from build123d import *

# Parameters (mm, degrees)
SKETCH1_R           = 22
SKETCH1_R_2         = 20
BOSS_EXTRUDE1_DEPTH = 10
BOSS_EXTRUDE2_START = 100
SKETCH1_3_R         = 22
SKETCH1_3_R_2       = 20
BOSS_EXTRUDE2_DEPTH = 100
FILLET1_R           = 5
FILLET2_R           = 5
BOSS_EXTRUDE3_DEPTH = 2
CHAMFER1_SIZE       = 2.5
CHAMFER1_SIZE_2     = 6.868693549


with BuildPart() as part:
    # Sketch1 → Boss-Extrude1 (new body)
    # profile 1 of 2: a face of its own
    with BuildSketch(Plane(origin=(0, 0, 0), x_dir=(1, 0, 0), z_dir=(0, 1, 0))):
        with Locations(Location((0, 0, 0), (0, 0, 270))):
            Circle(SKETCH1_R)
        Circle(SKETCH1_R_2, mode=Mode.SUBTRACT)
    # profile 2 of 2: a face of its own
    with BuildSketch(Plane(origin=(0, 0, 0), x_dir=(1, 0, 0), z_dir=(0, 1, 0))):
        Circle(SKETCH1_R_2)
    extrude(amount=-BOSS_EXTRUDE1_DEPTH)

    # Sketch1<3> → Boss-Extrude2 (add)
    with BuildSketch(Plane(origin=(0, 0, 0), x_dir=(1, 0, 0), z_dir=(0, 1, 0)).offset(BOSS_EXTRUDE2_START)):
        with Locations(Location((0, 0, 0), (0, 0, 270))):
            Circle(SKETCH1_3_R)
        with Locations(Location((0, 0, 0), (0, 0, 270))):
            Circle(SKETCH1_3_R_2, mode=Mode.SUBTRACT)
    extrude(amount=-BOSS_EXTRUDE2_DEPTH)

    # Fillet1
    fillet1_edges = [part.edges().sort_by_distance(p)[0] for p in [
        (0, 0, -20),
    ]]
    fillet(fillet1_edges, radius=FILLET1_R)

    # Fillet2
    fillet2_edges = [part.edges().sort_by_distance(p)[0] for p in [
        (0, -10, -22),
    ]]
    fillet(fillet2_edges, radius=FILLET2_R)

    # Sketch2 → Boss-Extrude3 (add)
    with BuildSketch(Plane.XZ.offset(10)):
        with BuildLine():
            ThreePointArc((2.165063509, 10.75), (0, 12), (-2.165063509, 10.75))
            Line((-2.165063509, 10.75), (-2.5, 10.169872981))
            Line((-2.5, 10.169872981), (-2.5, 0))
            ThreePointArc((-2.5, 0), (0, -2.5), (2.5, 0))
            Line((2.5, 0), (2.5, 10.169872981))
            Line((2.5, 10.169872981), (2.165063509, 10.75))
        make_face()
        with BuildLine():
            ThreePointArc((-2.165063509, -4.75), (-2.5, -6), (-2.165063509, -7.25))
            Line((-2.165063509, -7.25), (2.165063509, -7.25))
            ThreePointArc((2.165063509, -7.25), (2.5, -6), (2.165063509, -4.75))
            Line((2.165063509, -4.75), (-2.165063509, -4.75))
        make_face()
    extrude(amount=BOSS_EXTRUDE3_DEPTH)

    # Chamfer1
    # the kernel refuses this chamfer: 6.868693549, 2.5 mm, written as the material it takes off along each edge
    with BuildSketch(Plane(origin=(0, 100, 0), x_dir=(0, 0, 1), z_dir=(-1, 0, 0))) as chamfer1_piece_1:
        Polygon((20 + CHAMFER1_SIZE, 0), (20, -CHAMFER1_SIZE_2), (20, 0), align=None)
    revolve(axis=Axis((0, 100, 0), (0, 1, 0)), mode=Mode.SUBTRACT)


solid = part.part
Build history of the part. All positions in model axes, mm. A direction names the side the tool comes from. Coordinates: 2 decimals unless noted, no trailing zeros. Order: outer loops, then holes, each group sorted by start corner. A loop starts at its lowest first (then second) coordinate and runs counter-clockwise, first axis right, second up. Notation, with made-up numbers: (54.5, 47.25) - (78.5, 47.25) arc R37 cw to (78.5, 85.25) - close; hole circle Ø2 at (-15, 28). An arc over 180 degrees is marked (long way). Write item = value, one per line. Start each with the question number.
1) Saw through at C-C on y = -3. Write the cut outline in (x, z).
2) Wall check: line 1 along X through (y, z) = (66.5, 0); line 2 along Y through (x, z) = (2, 0.5); line 3 along Y through (x, z) = (-10.5, 1.5). Give the ranges that are in metal, low to high. Write a range as from..to.
3) Saw through at A-A on y = 14. Write the cut outline in (x, z).
4) Two-plate mould, pull along Z, no slides. Class faces 5 (the face through (0, -12, 5)), 6 (the face through (-19.524, 49.683, -4.336)), 7 (the face through (0, -11, -7.25)): pulls with the +Z half, pulls with the -Z half, needs draft (parallel to the pull), parting line crosses it, or undercut.
5) Saw through at B-B on x = 0. Write the cut outline in (y, z), then the cut area to 3 significant figures.
6) 3-axis set-ups, long thin cutter, end or side, ignore diameter. For faces 1 (the face through (0, -11, 12)), 2 (the face through (0, 0, 0)), 3 (the face through (0, -11, -4.75)), 4 (the face through (-2.5, -11, -6)): which of +Z, -Z, +X, -X, +Y, -Y reach the whole face in a straight line?
7) Flat gauge pins, fed straight in: pin 1 Ø4 at (x, z) = (-11.5, 3) entering from +Y; pin 2 Ø1.6 at (y, z) = (-11, 6.5) entering from -X; pin 3 Ø1 at (x, y) = (0, -11.5) entering from -Z. Where does each tip first touch, or does it go through?
From the geometry:
q1.outline = circle Ø44 at (0, 0)
q2.line_1 = -22..-20, 20..22
q2.line_2 = -12..0
q2.line_3 = -10..0
q3.outline = circle Ø44 at (0, 0); hole circle Ø40 at (0, 0)
q4.face_5 = needs draft
q4.face_6 = undercut
q4.face_7 = pulls with the -Z half
q5.outline = (-12, -7.25) - (-10, -7.25) - (-10, -17) arc R5 ccw to (-5, -22) - (98.63, -22) - (93.13, -20) - (5, -20) arc R5 cw to (0, -15) - (0, 15) arc R5 cw to (5, 20) - (93.13, 20) - (98.63, 22) - (-5, 22) arc R5 ccw to (-10, 17) - (-10, 12) - (-12, 12) - (-12, -2.5) - (-10, -2.5) - (-10, -4.75) - (-12, -4.75) - close
q5.area = 858 mm^2
q6.face_1 = +Z, -Y
q6.face_2 = +Y
q6.face_3 = +X, -X, -Y
q6.face_4 = -X, -Y
q7.pin_1 = 0
q7.pin_2 = -2.5
q7.pin_3 = -7.25
